The listing builds one solid part. Answer for the finished solid, in the listing's coordinates (mm). A direction names the side the tool comes from. Round coordinates to 2 decimals unless told otherwise and drop trailing zeros. Order: outer loops, then holes, each group sorted by start corner. A loop starts at its lowest first (then second) coordinate and runs counter-clockwise, first axis right, second up. Notation, with made-up numbers: (-33.5, 68.5) -> (18.5, 68.5) arc R31 cw to (18.5, 96.5) -> close; hole circle Ø4 at (27, 18.25). An arc over 180 degrees is marked (long way). Return JSON: item names as keys, results as strings. Group by question number.
(1) Consider line 1 (Y direction, x = 0, z = 2.75); line 2 (X direction, y = 31, z = 0); line 3 (X direction, y = 32, z = -26.5). Determine where each line is inside the solid, lowest interval first. Write a range as [from, to].
(2) The part is cut by section C-C (y = 29). Determine the outline of the cut face in (x, z), plus the area to 3 significant figures.
(3) The part is cut by section A-A (z = 0). Determine the outline of the cut face in (x, y).
(4) The part is cut by section B-B (x = 18). Determine the outline of the cut face in (y, z), plus the area to 3 significant figures.
(5) Which of the six approach directions +Z, -Z, +X, -X, +Y, -Y give full straight-line access (tool end or side, diameter ignored) to faces 5 (the face through (7, 28.9, -13.5)), 6 (the face through (-9, 27, -28)), 7 (the face through (-22.32, 46.17, -1.63))?
(6) Determine the mould class of faces 1 (the face through (-3.022, 48.771, 3.105)), 2 (the face through (-7, 29, -28)), 3 (the face through (25, 29, 0)), 4 (the face through (0, 29, -35.5)) for opening direction X: +X half, -X half, draft (parallel to the pull), parting line (faces both ways), or undercut.
(7) The part is cut by section D-D (z = -23). Determine the outline of the cut face in (x, y).
(8) Each of these flat-tipped pins is pushed along its axis until it touches: pin 1 (2 mm diameter, centred on x = -6.5, z = -21.5, fed in from -Y); pin 2 (14.5 mm diameter, centred on x = -15, z = 0, fed in from +Y); pin 3 (7.5 mm diameter, centred on x = -17, z = -3, fed in from -Y). Where does it stop, or does it pass through?
from build123d import *

# Parameters (mm, degrees)
SKETCH1_W           = 50
SKETCH1_H           = 21
BOSS_EXTRUDE1_DEPTH = 58
SKETCH3_R           = 7.5
CUT_EXTRUDE1_DEPTH  = 24
CUT_EXTRUDE2_REACH  = 66.025
SKETCH4_R           = 5
CUT_EXTRUDE3_START  = -24
SKETCH5_R           = 7.5
CUT_EXTRUDE3_DEPTH  = 24
CUT_EXTRUDE4_REACH  = 66.025
SKETCH6_R           = 4.5
CUT_EXTRUDE5_REACH  = 68.558
SKETCH8_W           = 10
SKETCH8_H           = 18
SKETCH7_R           = 4.1
CUT_EXTRUDE6_DEPTH  = 15
BOSS_EXTRUDE2_DEPTH = 25
SKETCH12_W          = 18
SKETCH12_H          = 20
BOSS_EXTRUDE3_DEPTH = 4
CUT_EXTRUDE7_DEPTH  = 78.975957833


with BuildPart() as part:
    # Sketch1 → Boss-Extrude1 (new body)
    with BuildSketch(Plane(origin=(0, 0, 0), x_dir=(1, 0, 0), z_dir=(0, 1, 0))):
        Rectangle(SKETCH1_W, SKETCH1_H)
    extrude(amount=BOSS_EXTRUDE1_DEPTH)

    # Sketch3 → Cut-Extrude1 (cut)
    with BuildSketch(Plane(origin=(0, 58, 0), x_dir=(1, 0, 0), z_dir=(0, 1, 0))):
        with Locations(Location((-15, 0, 0), (0, 0, 270))):
            Circle(SKETCH3_R)
    extrude(amount=-CUT_EXTRUDE1_DEPTH, mode=Mode.SUBTRACT)

    # Sketch4 → Cut-Extrude2 (cut, up to next)
    with BuildSketch(Plane(origin=(0, 58, 0), x_dir=(1, 0, 0), z_dir=(0, 1, 0)), mode=Mode.PRIVATE) as cut_extrude2_sk1:
        with Locations(Location((15, 0, 0), (0, 0, 270))):
            Circle(SKETCH4_R)
    cut_extrude2_tool1 = extrude(cut_extrude2_sk1.sketch, amount=-CUT_EXTRUDE2_REACH, mode=Mode.PRIVATE) & part.part
    add(cut_extrude2_tool1.solids().sort_by_distance((15, 58, 0))[0], mode=Mode.SUBTRACT)

    # Sketch5 → Cut-Extrude3 (cut)
    with BuildSketch(Plane.XZ.offset(CUT_EXTRUDE3_START)):
        with Locations(Location((-15, 0, 0), (0, 0, 90))):
            Circle(SKETCH5_R)
    extrude(amount=CUT_EXTRUDE3_DEPTH, mode=Mode.SUBTRACT)

    # Sketch6 → Cut-Extrude4 (cut, up to next)
    with BuildSketch(Plane.XZ, mode=Mode.PRIVATE) as cut_extrude4_sk1:
        with Locations(Location((-15, 0, 0), (0, 0, 270))):
            Circle(SKETCH6_R)
    cut_extrude4_tool1 = extrude(cut_extrude4_sk1.sketch, amount=-CUT_EXTRUDE4_REACH, mode=Mode.PRIVATE) & part.part
    add(cut_extrude4_tool1.solids().sort_by_distance((-15, 0, 0))[0], mode=Mode.SUBTRACT)

    # Sketch8 → Cut-Extrude5 (cut, up to next)
    with BuildSketch(Plane.XY.offset(10.5), mode=Mode.PRIVATE) as cut_extrude5_sk1:
        with Locations((0, 29)):
            Rectangle(SKETCH8_W, SKETCH8_H)
    cut_extrude5_tool1 = extrude(cut_extrude5_sk1.sketch, amount=-CUT_EXTRUDE5_REACH, mode=Mode.PRIVATE) & part.part
    add(cut_extrude5_tool1.solids().sort_by_distance((0, 29, 10.5))[0], mode=Mode.SUBTRACT)

    # Sketch7 → Cut-Extrude6 (cut)
    with BuildSketch(Plane.XY.offset(10.5)):
        with Locations((0, 46)):
            Circle(SKETCH7_R)
        with Locations(Location((0, 12, 0), (0, 0, 180))):
            Circle(SKETCH7_R)
    extrude(amount=-CUT_EXTRUDE6_DEPTH, mode=Mode.SUBTRACT)

    # Sketch11 → Boss-Extrude2 (add)
    with BuildSketch(Plane(origin=(0, 0, -10.5), x_dir=(-1, 0, 0), z_dir=(0, 0, -1))):
        Polygon((9, 19), (9, 39), (5, 39), (5, 38), (5, 20), (5, 19), align=None)
        Polygon((-9, 39), (-9, 19), (-5, 19), (-5, 20), (-5, 38), (-5, 39), align=None)
    extrude(amount=BOSS_EXTRUDE2_DEPTH)

    # Sketch12 → Boss-Extrude3 (add)
    with BuildSketch(Plane(origin=(0, 0, -35.5), x_dir=(-1, 0, 0), z_dir=(0, 0, -1))):
        with Locations((0, 29)):
            Rectangle(SKETCH12_W, SKETCH12_H)
    extrude(amount=BOSS_EXTRUDE3_DEPTH)

    # Sketch13 → Cut-Extrude7 (cut, through all)
    with BuildSketch(Plane(origin=(9, 0, 0), x_dir=(0, 0, -1), z_dir=(1, 0, 0))):
        with BuildLine():
            Line((16.25, 31.75), (25.25, 31.75))
            ThreePointArc((25.25, 31.75), (28, 29), (25.25, 26.25))
            Line((25.25, 26.25), (16.25, 26.25))
            ThreePointArc((16.25, 26.25), (13.5, 29), (16.25, 31.75))
        make_face()
    extrude(amount=-CUT_EXTRUDE7_DEPTH, mode=Mode.SUBTRACT)


solid = part.part
Answer below:
{
 "1": {"line 1": "y = [0, 7.9], [16.1, 20], [38, 41.9], [50.1, 58]", "line 2": "x = [-25, -19.5], [-10.5, -5], [5, 10], [20, 25]", "line 3": "x = [-9, -5], [5, 9]"},
 "2": {"outline": "(-25, -10.5) -> (-9, -10.5) -> (-9, -13.5) -> (-5, -13.5) -> (-5, 10.5) -> (-25, 10.5) -> close; (-9, -39.5) -> (9, -39.5) -> (9, -28) -> (5, -28) -> (5, -35.5) -> (-5, -35.5) -> (-5, -28) -> (-9, -28) -> close; (5, -13.5) -> (9, -13.5) -> (9, -10.5) -> (25, -10.5) -> (25, 10.5) -> (5, 10.5) -> close; hole circle Ø9 at (-15, 0); hole circle Ø10 at (15, 0)", "area": "854 mm²"},
 "3": {"outline": "(-25, 0) -> (-22.5, 0) -> (-22.5, 24) -> (-19.5, 24) -> (-19.5, 34) -> (-22.5, 34) -> (-22.5, 58) -> (-25, 58) -> close; (-10.5, 24) -> (-7.5, 24) -> (-7.5, 0) -> (10, 0) -> (10, 58) -> (-7.5, 58) -> (-7.5, 34) -> (-10.5, 34) -> close; (20, 0) -> (25, 0) -> (25, 58) -> (20, 58) -> close; hole (-5, 20) -> (5, 20) -> (5, 38) -> (-5, 38) -> close; hole circle Ø8.2 at (0, 12); hole circle Ø8.2 at (0, 46)"},
 "4": {"outline": "(0, -10.5) -> (58, -10.5) -> (58, -4) -> (0, -4) -> close; (0, 4) -> (58, 4) -> (58, 10.5) -> (0, 10.5) -> close", "area": "754 mm²"},
 "5": {"face 5": "+X, -X", "face 6": "-Z, -X, +Y, -Y", "face 7": "+Y"},
 "6": {"face 1": "undercut", "face 2": "draft", "face 3": "+X half", "face 4": "undercut"},
 "7": {"outline": "(-9, 19) -> (-5, 19) -> (-5, 26.25) -> (-9, 26.25) -> close; (-9, 31.75) -> (-5, 31.75) -> (-5, 39) -> (-9, 39) -> close; (5, 19) -> (9, 19) -> (9, 26.25) -> (5, 26.25) -> close; (5, 31.75) -> (9, 31.75) -> (9, 39) -> (5, 39) -> close"},
 "8": {"pin 1": "stops at y = 19", "pin 2": "stops at y = 34", "pin 3": "stops at y = 24"}
}
